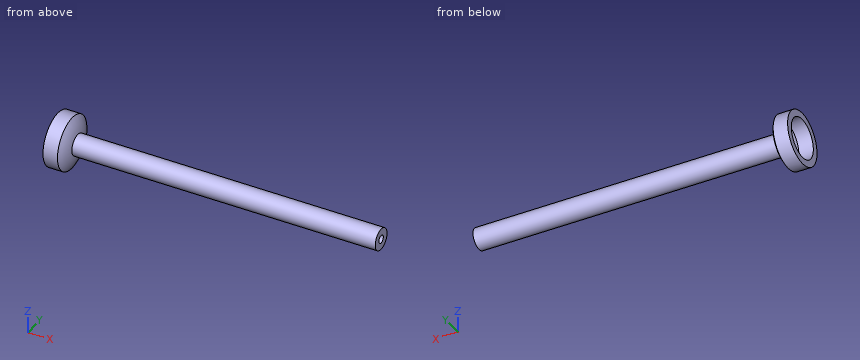
Autodesk Inventor part; units mm, degrees
ref_plane "YZ Plane" through (0, 0, 0) normal (1, 0, 0) x (0, 1, 0)
ref_plane "XZ Plane" through (0, 0, 0) normal (0, 1, 0) x (-1, 0, 0)
ref_plane "XY Plane" through (0, 0, 0) normal (0, 0, 1) x (1, 0, 0)
sketch "Sketch2" plane through (0, 0, 0) normal (0, 1, 0) x (-1, 0, 0)
  line L0 (-15, -3) -> (-165, -3)
  line L1 (-15, -8) -> (-165, -8)
  line L2 (146.5532, 0) -> (-237.9141, 0)
  line L3 (59.0935, -15) -> (59.0935, -20)
  line L4 (59.0935, -15) -> (48.2521, -15)
  line L5 (59.0935, -20) -> (48.2521, -20)
  arc A0 (44.0935, -3) -> (48.2521, -15) centre (91.6293, 6.7531) ccw
  arc A1 (44.0935, -8) -> (48.2521, -20) centre (72.6082, -4.8387) ccw
  line L6 (-165, -8) -> (-182.9902, -8)
  line L7 (-182.9902, -3) -> (-165, -3)
  line L8 (-182.9902, -8) -> (-182.9902, -3)
  line L9 (-15, -3) -> (5.213, -3)
  line L10 (-15, -8) -> (5.213, -8)
  line L11 (44.0935, -3) -> (5.213, -3)
  line L12 (5.213, -8) -> (44.0935, -8)
  point P0 (0, 0)
  point P1 (-13.1291, -22.6955)
  point P2 (-13.1263, -14.83)
revolve "Revolution2" add sketch "Sketch2" angle 360 about axis through (-10, 0, 0) along (1, 0, 0)
equation "\"BendRadius\" = Thickness"
equation "\"BendReliefWidth\" = Thickness"
equation "\"BendReliefDepth\" = 0.5 * Thickness"
equation "\"CornerReliefSize\" = 4 * Thickness"
equation "\"MinimumRemnant\" = 2 * Thickness"
equation "\"TransitionRadius\" = BendRadius"
equation "\"JacobiRadiusSize\" = BendRadius"
equation "\"GapSize\" = Thickness"
properties part number "Rubber pipe"
Could you check a few things on this model? Use its own coordinates, in mm. Round coordinates to 2 decimals unless told otherwise and drop trailing zeros. Loops run counter-clockwise (first coordinate to the right, second up) from the corner with the lowest first, then second, coordinate; pieces in that order, holes last. Notation, with made-up numbers: M 54,86.25 L 105,86.25 A29 cw 105,119.25 Z; hole C 46,42 d5. An arc over 180 degrees is marked long. Put each result on its own line as item: value.
Q1. I need wall thicknesses on probe 1 along Y at (x, z) = (-54.5, 0); probe 2 along Y at (x, z) = (19, 0); probe 3 along Z at (x, y) = (26, -1). Which ranges of each line are inside material? Lowest first, please.
Check result:
probe 1: -20 to -15, 15 to 20
probe 2: -8 to -3, 3 to 8
probe 3: -7.94 to -2.83, 2.83 to 7.94
Q2. Imagine slicing it at A-A (x = 141). Write out the boundary of the cut face in (y, z).
Check result:
outline: C 0,0 d16; hole C 0,0 d6
Q3. For pin 1 (2 mm diameter, centred on x = 74, z = -8, fed in from -Y); pin 2 (10 mm diameter, centred on x = 2.5, z = -11.5, fed in from +Y); pin 3 (18 mm diameter, centred on y = 0, z = 0, fed in from +X); pin 4 (12 mm diameter, centred on x = 34, z = 14.5, fed in from +Y), each with a flat end and sliding along its axis, tell me the tip position at first contact or that it passes through.
Check result:
pin 1: y = -3.87
pin 2: y = 4.66
pin 3: x = 182.99
pin 4: through
